Read the model definition and answer for the solid it produces. Units are mm, in the model's axes. A direction names the side the tool comes from. Round coordinates to 2 decimals unless told otherwise and drop trailing zeros. Loops run counter-clockwise (first coordinate to the right, second up) from the corner with the lowest first, then second, coordinate; pieces in that order, holes last. Notation, with made-up numbers: (68.25, -5) - (81.25, -5) arc R25 cw to (81.25, 15) - close; hole circle Ø5 at (18, 30.25). An arc over 180 degrees is marked (long way). Use CSV: the item, a comma, the result in double quotes. Start each with the question number.
1. Consider line 1 along Y through (x, z) = (43.85, 4.5); line 2 along Y through (x, z) = (15, 7.25); line 3 along Y through (x, z) = (45, 2.75). Determine where each line is inside the solid, lowest interval first.
2. A tool of negligible diameter and unlimited length cuts with its end or side. For faces 4 (the conical face through (12.49, 28.08, 11.86)), 5 (the flat face through (43, 96, 11)), from which of +Z, -Z, +X, -X, +Y, -Y can it reach the whole face along a straight path? Write none if from no direction.
3. Find section A-A (y = 20.5). Give the vertices of the cut face in (x, z), and give its area (3 significant figures).
4. Find section D-D (x = 50). Give the vertices of the cut face in (y, z), and give its area (3 significant figures).
5. Given pin 1 Ø20 at (x, y) = (43.85, 36) entering from +Z; pin 2 Ø17.5 at (x, y) = (37.5, 84.5) entering from -Z; pin 3 Ø4 at (x, y) = (59.35, 20.5) entering from +Z, each flat-ended and moving along its own axis, determine where each tip first touches the part or whether it passes through.
6. Determine the mould class of faces 1 (the flat face through (5, 81, 7)), 2 (the flat face through (35, 0, 7)), 3 (the cylindrical face through (59.155, 21.987, 6.743)) for opening direction X: +X half, -X half, draft (parallel to the pull), parting line (faces both ways), or undercut.
7. Find section C-C (y = 130). Give the vertices of the cut face in (x, z).
8. Find section B-B (x = 15). Give the vertices of the cut face in (y, z), and give its area (3 significant figures).
from build123d import *

# Parameters (mm, degrees)
SKIZZE1_W                        = 65
SKIZZE1_H                        = 160
AUFSATZ_LINEAR_AUSTRAGEN1_DEPTH  = 15
SKIZZE2_R                        = 17.5
SCHNITT_LINEAR_AUSTRAGEN1_DEPTH  = 11
SKIZZE4_R                        = 15.25
SCHNITT_LINEAR_AUSTRAGEN3_DEPTH  = 10
SKIZZE5_R                        = 11
SCHNITT_LINEAR_AUSTRAGEN4_DEPTH  = 20
SKIZZE7_R                        = 3
SCHNITT_LINEAR_AUSTRAGEN6_DEPTH  = 17
FASE1_SIZE                       = 3.3
SKIZZE10_R                       = 3
SCHNITT_LINEAR_AUSTRAGEN9_DEPTH  = 29
FASE2_SIZE                       = 3.3
SKIZZE11_R                       = 1.5
SCHNITT_LINEAR_AUSTRAGEN10_DEPTH = 44
FASE3_SIZE                       = 1.7
SKIZZE13_R                       = 4
SCHNITT_LINEAR_AUSTRAGEN12_DEPTH = 35
SKIZZE14_W                       = 15
SKIZZE14_H                       = 160
SCHNITT_LINEAR_AUSTRAGEN13_DEPTH = 5


with BuildPart() as part:
    # Skizze1 → Aufsatz-Linear austragen1 (new body)
    with BuildSketch(Plane.XY):
        with Locations((32.5, 80)):
            Rectangle(SKIZZE1_W, SKIZZE1_H)
    extrude(amount=AUFSATZ_LINEAR_AUSTRAGEN1_DEPTH)

    # Skizze2 → Schnitt-Linear austragen1 (cut)
    with BuildSketch(Plane(origin=(0, 0, 0), x_dir=(-1, 0, 0), z_dir=(0, 0, -1))):
        with Locations((-43.85, 80)):
            Circle(SKIZZE2_R)
    extrude(amount=-SCHNITT_LINEAR_AUSTRAGEN1_DEPTH, mode=Mode.SUBTRACT)

    # Skizze4 → Schnitt-Linear austragen3 (cut)
    with BuildSketch(Plane(origin=(0, 0, 11), x_dir=(-1, 0, 0), z_dir=(0, 0, -1))):
        with Locations((-43.85, 80)):
            Circle(SKIZZE4_R)
    extrude(amount=-SCHNITT_LINEAR_AUSTRAGEN3_DEPTH, mode=Mode.SUBTRACT)

    # Skizze5 → Schnitt-Linear austragen4 (cut)
    with BuildSketch(Plane.XY.offset(15)):
        with Locations((43.85, 36)):
            Circle(SKIZZE5_R)
    extrude(amount=-SCHNITT_LINEAR_AUSTRAGEN4_DEPTH, mode=Mode.SUBTRACT)

    # Skizze7 → Schnitt-Linear austragen6 (cut)
    with BuildSketch(Plane.XY.offset(15)):
        with Locations((15, 8)):
            Circle(SKIZZE7_R)
        with Locations((50, 8)):
            Circle(SKIZZE7_R)
    extrude(amount=-SCHNITT_LINEAR_AUSTRAGEN6_DEPTH, mode=Mode.SUBTRACT)

    # Fase1
    fase1_edges = [part.edges().sort_by_distance(p)[0] for p in [
        (12, 8, 15),
        (47, 8, 15),
    ]]
    chamfer(fase1_edges, length=FASE1_SIZE)

    # Skizze10 → Schnitt-Linear austragen9 (cut)
    with BuildSketch(Plane.XY.offset(15)):
        with Locations((15, 30)):
            Circle(SKIZZE10_R)
    extrude(amount=-SCHNITT_LINEAR_AUSTRAGEN9_DEPTH, mode=Mode.SUBTRACT)

    # Fase2
    fase2_edges = [part.edges().sort_by_distance(p)[0] for p in [
        (12, 30, 15),
    ]]
    chamfer(fase2_edges, length=FASE2_SIZE)

    # Skizze11 → Schnitt-Linear austragen10 (cut)
    with BuildSketch(Plane.XY.offset(15)):
        with Locations((59.35, 51.5)):
            Circle(SKIZZE11_R)
        with Locations((59.35, 20.5)):
            Circle(SKIZZE11_R)
        with Locations((28.35, 51.5)):
            Circle(SKIZZE11_R)
        with Locations((28.35, 20.5)):
            Circle(SKIZZE11_R)
    extrude(amount=-SCHNITT_LINEAR_AUSTRAGEN10_DEPTH, mode=Mode.SUBTRACT)

    # Fase3
    fase3_edges = [part.edges().sort_by_distance(p)[0] for p in [
        (57.85, 51.5, 15),
        (57.85, 20.5, 15),
        (26.85, 51.5, 15),
        (26.85, 20.5, 15),
    ]]
    chamfer(fase3_edges, length=FASE3_SIZE)

    # Skizze13 → Schnitt-Linear austragen12 (cut)
    with BuildSketch(Plane.XY.offset(15)):
        with Locations((43.85, 130)):
            Circle(SKIZZE13_R)
    extrude(amount=-SCHNITT_LINEAR_AUSTRAGEN12_DEPTH, mode=Mode.SUBTRACT)

    # Skizze14 → Schnitt-Linear austragen13 (cut)
    with BuildSketch(Plane.ZY):
        with Locations((7.5, 80)):
            Rectangle(SKIZZE14_W, SKIZZE14_H)
    extrude(amount=-SCHNITT_LINEAR_AUSTRAGEN13_DEPTH, mode=Mode.SUBTRACT)


solid = part.part
Filled sheet:
1,line 1,"y = 0 to 25, 47 to 62.5, 97.5 to 126, 134 to 160"
1,line 2,"y = 0 to 5, 11 to 27, 33 to 160"
1,line 3,"y = 0 to 25.06, 46.94 to 62.54, 97.46 to 126.17, 133.83 to 160"
2,face 4,"+Z"
2,face 5,"-Z"
3,outline,"(5, 0) - (26.85, 0) - (26.85, 13.3) - (25.15, 15) - (5, 15) - close; (29.85, 0) - (57.85, 0) - (57.85, 13.3) - (56.15, 15) - (31.55, 15) - (29.85, 13.3) - close; (60.85, 0) - (65, 0) - (65, 15) - (62.55, 15) - (60.85, 13.3) - close"
3,area,"804 mm²"
4,outline,"(0, 0) - (5, 0) - (5, 11.7) - (1.7, 15) - (0, 15) - close; (11, 0) - (26.88, 0) - (26.88, 15) - (14.3, 15) - (11, 11.7) - close; (45.12, 0) - (63.62, 0) - (63.62, 11) - (66.05, 11) - (66.05, 15) - (45.12, 15) - close; (93.95, 11) - (96.38, 11) - (96.38, 0) - (160, 0) - (160, 15) - (93.95, 15) - close"
4,area,"1,550 mm²"
5,pin 1,"passes through"
5,pin 2,"stops at z = 11"
5,pin 3,"stops at z = 13.8"
6,face 1,"-X half"
6,face 2,"draft"
6,face 3,"undercut"
7,outline,"(5, 0) - (39.85, 0) - (39.85, 15) - (5, 15) - close; (47.85, 0) - (65, 0) - (65, 15) - (47.85, 15) - close"
8,outline,"(0, 0) - (5, 0) - (5, 11.7) - (1.7, 15) - (0, 15) - close; (11, 0) - (27, 0) - (27, 11.7) - (23.7, 15) - (14.3, 15) - (11, 11.7) - close; (33, 0) - (160, 0) - (160, 15) - (36.3, 15) - (33, 11.7) - close"
8,area,"2,200 mm²"
